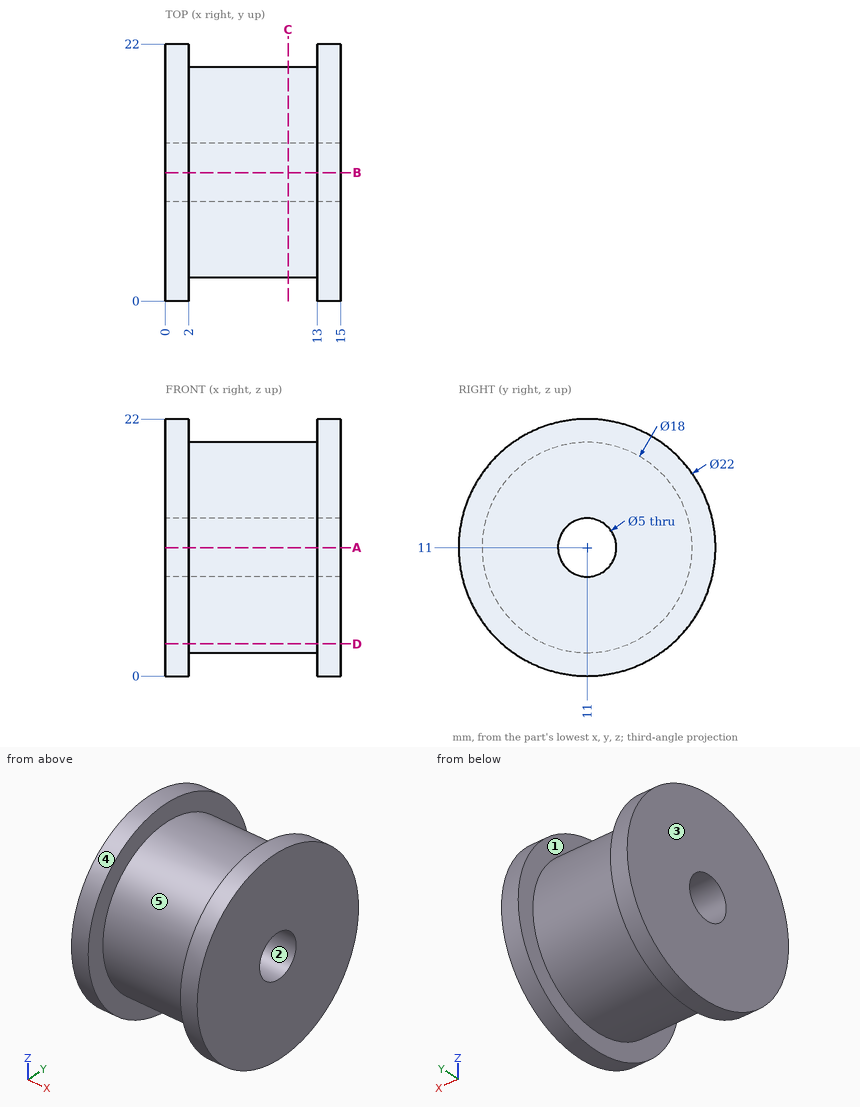
Answer from the drawing. Dimensions are ordinates in mm from the lowest x, y and z of the part. A direction names the side the tool comes from. Round coordinates to 2 decimals unless told otherwise and drop trailing zeros. Loops run counter-clockwise (first coordinate to the right, second up) from the corner with the lowest first, then second, coordinate; pieces in that order, holes last.
Q1. Which of the six approach directions +Z, -Z, +X, -X, +Y, -Y give full straight-line access (tool end or side, diameter ignored) to the marked faces 4 and 5?
Q2. Consider probe 1 along X at (y, z) = (17, 19.25); probe 2 along Y at (x, z) = (4, 11); probe 3 along Z at (x, y) = (7.25, 10). Determine where each line is inside the solid, lowest interval first.
Q3. Section A-A on z = 11 is taken. Write down the section's boundary in (x, y), and give its area (3 significant figures).
Q4. Section C-C on x = 10.5 is taken. Write down the section's boundary in (y, z).
Q5. Determine the mould class of the marked faces 1, 2 and 3 for opening direction X: released by +X, released by -X, zero draft, split by the parting line, or undercut.
Q6. Each of these flat-tipped pins is pushed along its axis until it touches: pin 1 (1.5 mm diameter, centred on x = 4.5, y = 3.5, fed in from -Z); pin 2 (3 mm diameter, centred on y = 11, z = 11, fed in from +X); pin 3 (5 mm diameter, centred on x = 2, y = 7, fed in from +Z); pin 4 (8 mm diameter, centred on x = 8, y = 17.5, fed in from -Z). Where does it stop, or does it pass through?
Q7. Section D-D on z = 2.75 is taken. Write down the section's boundary in (x, y).
Output:
1. face 4: +X, -X
1. face 5: none
2. probe 1: x = 0 to 2, 13 to 15
2. probe 2: y = 2 to 8.5, 13.5 to 20
2. probe 3: z = 2.06 to 8.71, 13.29 to 19.94
3. outline: (0, 0) - (2, 0) - (2, 2) - (13, 2) - (13, 0) - (15, 0) - (15, 8.5) - (0, 8.5) - close; (0, 13.5) - (15, 13.5) - (15, 22) - (13, 22) - (13, 20) - (2, 20) - (2, 22) - (0, 22) - close
3. area: 211 mm2
4. outline: circle Ø18 at (11, 11); hole circle Ø5 at (11, 11)
5. face 1: undercut
5. face 2: zero draft
5. face 3: released by -X
6. pin 1: stops at z = 5.05
6. pin 2: passes through
6. pin 3: stops at z = 21.9
6. pin 4: stops at z = 2.35
7. outline: (0, 3.72) - (2, 3.72) - (2, 7.4) - (13, 7.4) - (13, 3.72) - (15, 3.72) - (15, 18.28) - (13, 18.28) - (13, 14.6) - (2, 14.6) - (2, 18.28) - (0, 18.28) - close
